Part model, mm, in its own coordinate system. A direction names the side the tool comes from. Coordinates: 2 decimals unless noted, no trailing zeros. Loops run counter-clockwise (first coordinate to the right, second up) from the corner with the lowest first, then second, coordinate; pieces in that order, holes last. Notation, with made-up numbers: (-11, -16.5) - (16, -16.5) arc R20 cw to (16, -8.5) - close; hole circle Ø8 at (12.25, 83.5). An arc over 180 degrees is marked (long way). Use a Markdown table: item, result. Add a question column.
1) Band-saw the part on C-C (x = -4.95). Give the number of separate pieces and of enclosed holes in the cut face, plus the area to 3 significant figures.
2) Band-saw the part on B-B (z = -0.5). Give the cut face in (x, y), plus the area to 3 significant figures.
3) Band-saw the part on A-A (y = -0.25). Give the cut face in (x, z).
4) Tool access for faces 4 (the face through (-1.5, 2, 4)), 5 (the face through (-2.979, -8.428, -1.107)), 6 (the face through (-4.76, 7.45, 0.78)): list every direction of +Z, -Z, +X, -X, +Y, -Y with a clear straight run to the whole face (end or side of a thin tool).
5) Band-saw the part on D-D (z = 7). Give the cut face in (x, y).
6) Drop flat-ended pins along their axis: P1, Ø0.7, axis at x = -5, z = -2, coming from the +Y side; P2, Ø1.2, axis at x = -4.5, y = 7, coming from the -Z side; P3, Ø0.7, axis at x = -5, z = -1.5, coming from the -Y side. Give the stop position or say it passes through.
7) Pull direction X, two halves, no side cores. Call faces 1 (the face through (-5.5, 6, 1)), 2 (the face through (-4.76, 7.46, 1.42)), 3 (the face through (-1.5, 7.4, 4.5)): +X half, -X half, draft (parallel to the pull), parting line (faces both ways), or undercut.
8) Probe probe 1 along Y at (x, z) = (-1.2, 0); probe 2 along Y at (x, z) = (-3.8, 0); probe 3 along X at (y, z) = (5.5, -8). List the from-to ranges inside material, lowest first. Write a range as [from, to].
from build123d import *

# Parameters (mm, degrees)
SKETCH1_W          = 5
SKETCH1_H          = 5.9
SKETCH2_W          = 3
SKETCH2_H          = 1.5
SKETCH3_R          = 8
CUT_EXTRUDE1_DEPTH = 1.5
CUT_EXTRUDE2_DEPTH = 1.5


with BuildPart() as part:
    # Sketch1 → Revolve1 (revolve)
    with BuildSketch(Plane.XY, mode=Mode.PRIVATE) as revolve1_sk:
        with Locations((-3, 7.05)):
            Rectangle(SKETCH1_W, SKETCH1_H)
    revolve(revolve1_sk.sketch.rotate(Axis((0, 0, 0), (1, 0, 0)), 90), axis=Axis((0, 0, 0), (1, 0, 0)))

    # Sketch2 → Cut-Revolve1 (revolve, cut)
    with BuildSketch(Plane.XY, mode=Mode.PRIVATE) as cut_revolve1_sk:
        with Locations((-3, 9.25)):
            Rectangle(SKETCH2_W, SKETCH2_H)
    revolve(cut_revolve1_sk.sketch.rotate(Axis((0, 0, 0), (1, 0, 0)), 90), axis=Axis((0, 0, 0), (1, 0, 0)), mode=Mode.SUBTRACT)

    # Sketch3 → Cut-Extrude1 (cut)
    with BuildSketch(Plane(origin=(0, 0, 0), x_dir=(0, 0, -1), z_dir=(1, 0, 0))):
        Circle(SKETCH3_R)
    extrude(amount=-CUT_EXTRUDE1_DEPTH, mode=Mode.SUBTRACT)

    # Sketch5 → Cut-Extrude2 (cut)
    # profile 1 of 2: a face of its own
    with BuildSketch(Plane.ZY.offset(5.5)):
        Polygon((-1.793384415, 8.175), (-0.9125, 8.175), (-0.9125, 5), (-1.482371795, 5), (-1.482371795, 7.645833333), (-2.133653846, 7.645833333), align=None)
    # profile 2 of 2: a face of its own
    with BuildSketch(Plane.ZY.offset(5.5)):
        with BuildLine():
            Line((1.191446314, 8.256410256), (1.695808293, 8.00073117))
            Line((1.695808293, 8.00073117), (1.142472957, 6.913141026))
            add(Edge.make_bspline(
                [(1.142472957, 6.913141026), (1.175163489, 6.912294651), (1.239552854, 6.910627578), (1.334288739, 6.897154014), (1.424858008, 6.873861453), (1.512173869, 6.842987227), (1.595168965, 6.801522834), (1.675179981, 6.752198775), (1.750136991, 6.69204278), (1.821758695, 6.62539313), (1.886883941, 6.551554895), (1.943456732, 6.472213367), (1.99275892, 6.389298934), (2.031084458, 6.300956598), (2.061999112, 6.208650736), (2.084305396, 6.11201236), (2.097031755, 6.010761626), (2.098786295, 5.941977417), (2.099679487, 5.906961138)],
                knots=[0, 0, 0, 0, 1.013260694, 1.995783107, 2.958651975, 3.908806537, 4.861209129, 5.829647963, 6.817170299, 7.835534541, 8.860094905, 9.863329007, 10.853101798, 11.844815043, 12.84250023, 13.867713965, 14.914507806, 16, 16, 16, 16], degree=3))
            add(Edge.make_bspline(
                [(2.099679487, 5.906961138), (2.098842493, 5.873207569), (2.097188113, 5.806491238), (2.083512477, 5.708501914), (2.06141193, 5.614486889), (2.02982581, 5.524633922), (1.989677297, 5.438503809), (1.940578386, 5.356147091), (1.882121896, 5.278179194), (1.81581818, 5.205014401), (1.743336781, 5.138324152), (1.666937439, 5.079045977), (1.585972755, 5.030079955), (1.501973056, 4.988727002), (1.413391857, 4.957868741), (1.32155478, 4.934576099), (1.225765397, 4.921135234), (1.160746018, 4.91944503), (1.127844551, 4.918589744)],
                knots=[0, 0, 0, 0, 1.049934834, 2.075270938, 3.072134561, 4.05064612, 5.033440221, 6.024524368, 7.028587226, 8.060776465, 9.092543989, 10.090062252, 11.064205434, 12.031961459, 12.998029633, 13.977230324, 14.976426867, 16, 16, 16, 16], degree=3))
            add(Edge.make_bspline(
                [(1.127844551, 4.918589744), (1.093439615, 4.919291632), (1.025786964, 4.9206718), (0.926794204, 4.936126046), (0.831851626, 4.959390259), (0.741492825, 4.992607602), (0.655155886, 5.034903587), (0.57385727, 5.087240616), (0.496912148, 5.149041549), (0.42514087, 5.218915965), (0.360480297, 5.295453826), (0.302808469, 5.374920054), (0.254018029, 5.457439347), (0.214523305, 5.542923478), (0.183708605, 5.631100047), (0.162267859, 5.722136406), (0.148297235, 5.81579108), (0.146659497, 5.879350442), (0.145833333, 5.911413261)],
                knots=[0, 0, 0, 0, 1.063775006, 2.091769615, 3.092589432, 4.084662827, 5.064601646, 6.061867366, 7.070035304, 8.113879863, 9.156342271, 10.166834137, 11.149076039, 12.117706134, 13.076241869, 14.034148791, 15.008317125, 16, 16, 16, 16], degree=3))
            add(Edge.make_bspline(
                [(0.145833333, 5.911413261), (0.146269862, 5.936242164), (0.14714535, 5.986038176), (0.155943478, 6.060604999), (0.169319723, 6.135367552), (0.184824543, 6.198454562), (0.20078984, 6.251801232), (0.216859033, 6.296947076), (0.236773258, 6.347049092), (0.259538168, 6.40223522), (0.285869634, 6.462439071), (0.315630108, 6.527496544), (0.348893678, 6.597900304), (0.372615185, 6.646256786), (0.384975962, 6.671454327)],
                knots=[0, 0, 0, 0, 1.110454016, 2.227089276, 3.35462975, 4.507227546, 5.131400587, 5.845402449, 6.650387134, 7.543487832, 8.516250726, 9.590168902, 10.744287919, 12, 12, 12, 12], degree=3))
            Line((0.384975962, 6.671454327), (1.191446314, 8.256410256))
        make_face()
        with BuildLine():
            add(Edge.make_bspline(
                [(1.115124199, 6.383974359), (1.087780016, 6.382720139), (1.034271038, 6.380265795), (0.958189275, 6.354562713), (0.888819969, 6.314240974), (0.828689797, 6.258085155), (0.77839644, 6.190976745), (0.741439117, 6.114430641), (0.719207234, 6.029468327), (0.716897483, 5.970064094), (0.715705128, 5.939398037)],
                knots=[0, 0, 0, 0, 0.981744412, 1.921144944, 2.858899012, 3.85339082, 4.86292663, 5.863643845, 6.897155691, 8, 8, 8, 8], degree=3))
            add(Edge.make_bspline(
                [(0.715705128, 5.939398037), (0.717116914, 5.908721768), (0.719862931, 5.849054373), (0.742930763, 5.763283067), (0.780699961, 5.684998689), (0.833668853, 5.617000948), (0.895853571, 5.560557558), (0.964809047, 5.518814972), (1.039385079, 5.493171132), (1.090971142, 5.490042243), (1.117032252, 5.488461538)],
                knots=[0, 0, 0, 0, 1.098279937, 2.136227893, 3.159405121, 4.194678092, 5.206500211, 6.154139736, 7.067477469, 8, 8, 8, 8], degree=3))
            add(Edge.make_bspline(
                [(1.117032252, 5.488461538), (1.144555729, 5.490070396), (1.198534047, 5.493225646), (1.276401312, 5.51779044), (1.347533526, 5.558833701), (1.410428162, 5.615096382), (1.464453459, 5.682318178), (1.501833508, 5.761062388), (1.525967776, 5.847452761), (1.528499022, 5.908062449), (1.529807692, 5.939398037)],
                knots=[0, 0, 0, 0, 0.96921794, 1.900804717, 2.848419905, 3.844199796, 4.861108892, 5.867439427, 6.897452859, 8, 8, 8, 8], degree=3))
            add(Edge.make_bspline(
                [(1.529807692, 5.939398037), (1.528316878, 5.970046189), (1.525429742, 6.029399913), (1.503743929, 6.114760256), (1.465025374, 6.191011323), (1.41359409, 6.258362168), (1.351394556, 6.314492947), (1.279248949, 6.354880703), (1.199691644, 6.380220258), (1.143724347, 6.382704747), (1.115124199, 6.383974359)],
                knots=[0, 0, 0, 0, 1.083229974, 2.097801324, 3.086792542, 4.086858909, 5.079819718, 6.026392613, 6.991456328, 8, 8, 8, 8], degree=3))
        make_face(mode=Mode.SUBTRACT)
    extrude(amount=-CUT_EXTRUDE2_DEPTH, mode=Mode.SUBTRACT)


solid = part.part
Answer block:
| question | item | result |
|---|---|---|
| 1 | separate pieces | 2 |
| 1 | enclosed holes | 3 |
| 1 | area | 256 mm2 |
| 2 | outline | (-5.5, -9.99) - (-4.5, -9.99) - (-4.5, -8.49) - (-1.5, -8.49) - (-1.5, -9.99) - (-0.5, -9.99) - (-0.5, -7.98) - (-1.5, -7.98) - (-1.5, -4.07) - (-5.5, -4.07) - close; (-5.5, 4.07) - (-1.5, 4.07) - (-1.5, 7.98) - (-0.5, 7.98) - (-0.5, 9.99) - (-1.5, 9.99) - (-1.5, 8.49) - (-4.5, 8.49) - (-4.5, 9.99) - (-5.5, 9.99) - close |
| 2 | area | 42.3 mm2 |
| 3 | outline | (-5.5, -10) - (-4.5, -10) - (-4.5, -8.5) - (-1.5, -8.5) - (-1.5, -10) - (-0.5, -10) - (-0.5, -8) - (-1.5, -8) - (-1.5, -4.09) - (-5.5, -4.09) - close; (-5.5, 4.09) - (-1.5, 4.09) - (-1.5, 8) - (-0.5, 8) - (-0.5, 10) - (-1.5, 10) - (-1.5, 8.5) - (-4.5, 8.5) - (-4.5, 10) - (-5.5, 10) - close |
| 4 | face 4 | +X |
| 4 | face 5 | none |
| 4 | face 6 | -X |
| 5 | outline | (-5.5, -7.14) - (-4.5, -7.14) - (-4.5, -4.82) - (-1.5, -4.82) - (-1.5, -7.14) - (-0.5, -7.14) - (-0.5, -3.87) - (-1.5, -3.87) - (-1.5, 3.87) - (-0.5, 3.87) - (-0.5, 7.14) - (-1.5, 7.14) - (-1.5, 4.82) - (-4.5, 4.82) - (-4.5, 7.14) - (-5.5, 7.14) - close |
| 6 | P1 | y = 9.86 |
| 6 | P2 | z = -7.68 |
| 6 | P3 | y = -9.93 |
| 7 | face 1 | -X half |
| 7 | face 2 | draft |
| 7 | face 3 | undercut |
| 8 | probe 1 | [-10, -8], [8, 10] |
| 8 | probe 2 | [-8.5, -4.1], [4.1, 8.5] |
| 8 | probe 3 | [-5.5, -4.5], [-1.5, -0.5] |
